Autodesk Fusion 360 part; units mm, degrees
sketch "Sketch1" plane through (0, 0, 0) normal (0, 0, 1) x (1, 0, 0)
  circle A0 centre (0, 0) radius 31.9
  line L0 (0, 0) -> (-31.9, 0) construction
  line L1 (0, 0) -> (31.9, 0) construction
  circle A1 centre (23.029, 0) radius 1.75
  circle A2 centre (-23.029, 0) radius 1.75
  circle A3 centre (-23.029, 0) radius 3
  circle A4 centre (23.029, 0) radius 3
  circle A5 centre (0, 0) radius 4
  dimension "d1" = 63.8
  dimension "d2" = 3.5
  dimension "d3" = 23.029
  dimension "d4" = 3.5
  dimension "d5" = 23.029
  dimension "d6" = 6
  dimension "d7" = 6
  dimension "d8" = 8
extrude "Extrude1" add sketch "Sketch1" along normal blind 3 contours A0 | A3 | A4 | A5
extrude "Extrude3" add sketch "Sketch1" against normal blind 12 contours A5
fillet "Fillet2" radius 3 1 edges at (-3.7293, -1.4465, 0)
chamfer "Chamfer2" distance 1.25 angle 45 2 edges at (21.3974, 0.6328, 0) (-24.6606, 0.6328, 0)
Can you work these out from the model? Positions are in its coordinate system, mm. A direction names the side the tool comes from. Coordinates: 2 decimals unless noted, no trailing zeros. Write each loop counter-clockwise with the first axis right and the second up, starting at its lowest first coordinate (ties: lowest second). Pieces come first, ordered by that corner, then holes. Notation, with made-up numbers: M 56.25,19 L 75.25,19 A9 cw 75.25,36 Z; hole C -31,31 d1. An arc over 180 degrees is marked long. Answer as CSV lines item,"result".
Item 1: Imagine slicing it at D-D on y = 19. List the corners of the cut face in (x, z) for me, plus the area to 3 significant figures.
Geometry results:
outline,"M -25.62,0 L 25.62,0 L 25.62,3 L -25.62,3 Z"
area,"154 mm2"
Item 2: Imagine slicing it at B-B on x = 0. List the corners of the cut face in (y, z) for me, plus the area to 3 significant figures.
Geometry results:
outline,"M -31.9,0 L -7,0 A3 cw -4,-3 L -4,-12 L 4,-12 L 4,-3 A3 cw 7,0 L 31.9,0 L 31.9,3 L -31.9,3 Z"
area,"291 mm2"
Item 3: We'd pull the mould along Y, two halves only. Please class faces 1 (the cylindrical face through (30.427, -9.582, 1.479)), 2 (the conical face through (23, 2, 1)), 3 (the flat face through (0, 0, 3)): +Y half, -Y half, draft (parallel to the pull), parting line (faces both ways), or undercut.
Geometry results:
face 1,"parting line"
face 2,"undercut"
face 3,"draft"
Item 4: Imagine slicing it at A-A on y = 0. List the corners of the cut face in (x, z) for me, plus the area to 3 significant figures.
Geometry results:
outline,"M -31.9,0 L -26.03,0 L -24.78,1.25 L -24.78,3 L -31.9,3 Z; M -21.28,1.25 L -20.03,0 L -7,0 A3 cw -4,-3 L -4,-12 L 4,-12 L 4,-3 A3 cw 7,0 L 20.03,0 L 21.28,1.25 L 21.28,3 L -21.28,3 Z; M 24.78,1.25 L 26.03,0 L 31.9,0 L 31.9,3 L 24.78,3 Z"
area,"267 mm2"
Item 5: On a 3-axis mill with a long thin cutter (end or side, diameter ignored), from which of +Z, -Z, +X, -X, +Y, -Y can I reach the whole of each face in a straight line? I mean faces 4 (the cylindrical face through (-0.867, -3.905, -7.437)), 5 (the cylindrical face through (-24.777, -0.077, 2.113)). Say none if no direction works.
Geometry results:
face 4,"-Z"
face 5,"+Z, -Z"
Item 6: Please list where these lines run through material, in increasing order: line 1 along Z through (x, y) = (-11, 0); line 2 along Y through (x, z) = (5.5, 1); line 3 along Y through (x, z) = (-7, 0.25).
Geometry results:
line 1,"z = 0 to 3"
line 2,"y = -31.42 to 31.42"
line 3,"y = -31.12 to 31.12"
Item 7: I'm going to push flat-ended pins straight in: P1, Ø3, axis at x = -19, y = 12.5, coming from the -Z side; P2, Ø4.5, axis at x = 23.029, y = 0, coming from the +Z side; P3, Ø1.5, axis at x = 0.5, z = -7, coming from the -Y side; P4, Ø4, axis at y = 4.5, z = 0, coming from the +X side. Where does each tip first touch, or does it pass through?
Geometry results:
P1,"stops at z = 0"
P2,"stops at z = 3"
P3,"stops at y = -4"
P4,"stops at x = 31.8"
Item 8: Imagine slicing it at C-C on z = -5.25. List the corners of the cut face in (x, y) for me, plus the area to 3 significant figures.
Geometry results:
outline,"C 0,0 d8"
area,"50.3 mm2"
